For this review, take the finished solid that the model builds, in its own axes (mm). A direction names the side the tool comes from. Give positions to 0.01 mm unless a question says otherwise; leave off trailing zeros. Order: outer loops, then holes, each group sorted by start corner. A loop starts at its lowest first (then second) coordinate and runs counter-clockwise, first axis right, second up.
from build123d import *

# Parameters (mm, degrees)
SKETCH1_R           = 34.925
BOSS_EXTRUDE1_DEPTH = 6.35
SKETCH2_W           = 3.81
SKETCH2_H           = 19.05
BOSS_EXTRUDE2_DEPTH = 44.45
SKETCH3_R           = 6.35
BOSS_EXTRUDE3_DEPTH = 25.4


with BuildPart() as part:
    # Sketch1 → Boss-Extrude1 (new body)
    with BuildSketch(Plane(origin=(0, 0, 0), x_dir=(1, 0, 0), z_dir=(0, 1, 0))):
        Circle(SKETCH1_R)
    extrude(amount=BOSS_EXTRUDE1_DEPTH)

    # Sketch2 → Boss-Extrude2 (add)
    with BuildSketch(Plane(origin=(0, 6.35, 0), x_dir=(1, 0, 0), z_dir=(0, 1, 0))):
        with Locations((-14.605, 0)):
            Rectangle(SKETCH2_W, SKETCH2_H)
        with Locations((14.605, 0)):
            Rectangle(SKETCH2_W, SKETCH2_H)
    extrude(amount=BOSS_EXTRUDE2_DEPTH)

    # Sketch3 → Boss-Extrude3 (add)
    with BuildSketch(Plane(origin=(-12.7, 0, 0), x_dir=(0, 0, -1), z_dir=(1, 0, 0))):
        with Locations((0, 44.45)):
            Circle(SKETCH3_R)
    extrude(amount=BOSS_EXTRUDE3_DEPTH)


solid = part.part
1) Clearance check with flat-ended pins moving along their axes: pin 1 (5.5 mm diameter, centred on y = 22.5, z = -2, fed in from +X); pin 2 (5 mm diameter, centred on x = -27, z = -18, fed in from +Y); pin 3 (12 mm diameter, centred on y = 15.5, z = 17.5, fed in from -X); pin 4 (3 mm diameter, centred on x = 11.5, z = -1, fed in from +Y). State where each tip first meets the part, or that it passes through.
Answer sheet:
pin 1: stops at x = 16.51
pin 2: stops at y = 6.35
pin 3: passes through
pin 4: stops at y = 50.8
2) We need section A-A on y = 27.5. Give the boundary of the cut face in (x, z) (3 decimals), then the cut area to 3 significant figures.
Answer sheet:
outline: (-16.51, -9.525) - (-12.7, -9.525) - (-12.7, 9.525) - (-16.51, 9.525) - close; (12.7, -9.525) - (16.51, -9.525) - (16.51, 9.525) - (12.7, 9.525) - close
area: 145 mm2
3) Tool access review of faces 5 (the face through (-0.178, 50.746, 0.827)), 6 (the face through (15, 28, -9.525)), 7 (the face through (-15, 28, 9.525)): name each direction out of +Z, -Z, +X, -X, +Y, -Y from which nothing blocks a thin tool from reaching the whole face with its end or side.
Answer sheet:
face 5: none
face 6: -Z, +X, -X, +Y
face 7: +Z, +X, -X, +Y
4) We need section B-B on x = 0. Give the boundary of the cut face in (y, z) (3 decimals).
Answer sheet:
outline: (0, -34.925) - (6.35, -34.925) - (6.35, 34.925) - (0, 34.925) - close; circle Ø12.7 at (44.45, 0)
5) To check wall thickness, follow line 1 (X direction, y = 26, z = 3); line 2 (Y direction, x = 10, z = -10); line 3 (Z direction, x = -13.5, y = 11.5) (3 decimals). State the ranges of each line that lie inside material, in increasing order.
Answer sheet:
line 1: x = -16.51 to -12.7, 12.7 to 16.51
line 2: y = 0 to 6.35
line 3: z = -9.525 to 9.525
6) Draft analysis for pull direction Y (two halves, no side actions). For faces 1 (the face through (12.7, 23, 0)), 2 (the face through (15, 50.8, 0)), 3 (the face through (0, 0, 0)), 4 (the face through (-27.715, 3.131, 21.251)), state which applies: +Y half, -Y half, draft (parallel to the pull), parting line (faces both ways), or undercut.
Answer sheet:
face 1: undercut
face 2: +Y half
face 3: -Y half
face 4: draft
7) We need section D-D on z = 2. Give the boundary of the cut face in (x, y).
Answer sheet:
outline: (-34.87, 0) - (34.87, 0) - (34.87, 6.35) - (16.51, 6.35) - (16.51, 50.8) - (12.7, 50.8) - (12.7, 50.48) - (-12.7, 50.48) - (-12.7, 50.8) - (-16.51, 50.8) - (-16.51, 6.35) - (-34.87, 6.35) - close; hole (-12.7, 6.35) - (12.7, 6.35) - (12.7, 38.42) - (-12.7, 38.42) - close
8) We need section C-C on y = 44.45. Give the boundary of the cut face in (x, z) (3 decimals).
Answer sheet:
outline: (-16.51, -9.525) - (-12.7, -9.525) - (-12.7, -6.35) - (12.7, -6.35) - (12.7, -9.525) - (16.51, -9.525) - (16.51, 9.525) - (12.7, 9.525) - (12.7, 6.35) - (-12.7, 6.35) - (-12.7, 9.525) - (-16.51, 9.525) - close
